Could you check a few things on this drawing? It's one solid part, dimensions in mm from its lowest x, y, z. Give positions to 0.01 mm unless a question says otherwise; leave off trailing zeros. Write each loop counter-clockwise with the first axis right and the second up, starting at its lowest first coordinate (ties: lowest second). Pieces come first, ordered by that corner, then holes.
1. Suppose I cut it at B-B (y = 74). Please give me the cut outline in (x, z).
2. If I drill on probe 1 along X at (y, z) = (28, 3); probe 2 along Y at (x, z) = (65.5, 5.25); probe 3 along X at (y, z) = (24, 3), over which ranges is the centre line in solid material (lowest first)?
3. I'm going to push flat-ended pins straight in: pin 1 (1.9 mm diameter, centred on y = 3, z = 2.5, fed in from +X); pin 2 (1.9 mm diameter, centred on y = 2.5, z = 3, fed in from -X); pin 3 (3 mm diameter, centred on y = 13, z = 3.5, fed in from -X). Where does each tip first touch, or does it pass through?
4. Suppose I cut it at A-A (x = 123). Please give me the cut outline in (y, z).
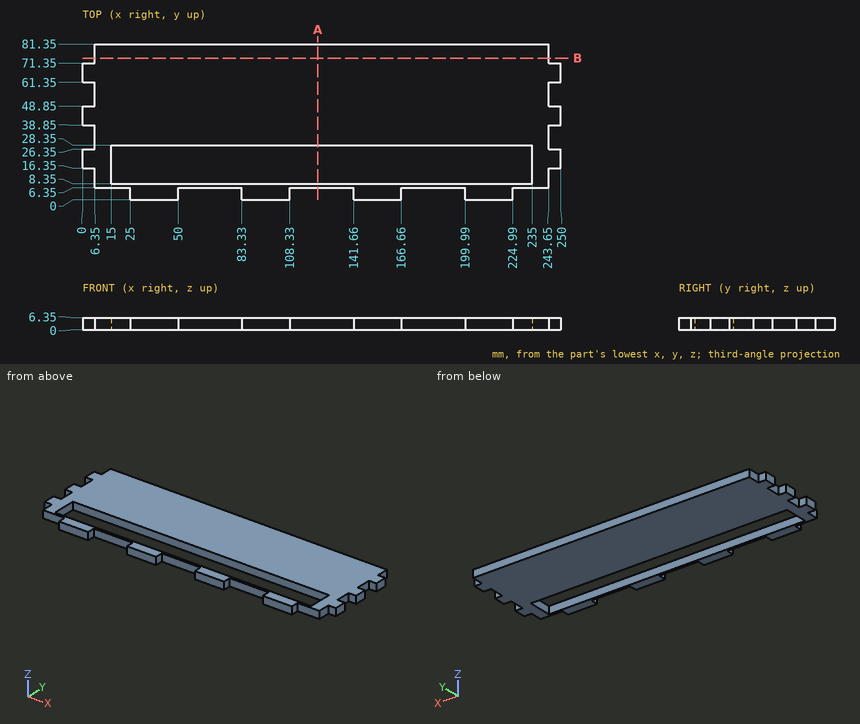
Checks:
1. outline: (6.35, 0) - (243.65, 0) - (243.65, 6.35) - (6.35, 6.35) - close
2. probe 1: x = 6.35 to 15, 235 to 243.65
2. probe 2: y = 6.35 to 8.35, 28.35 to 81.35
2. probe 3: x = 0 to 15, 235 to 250
3. pin 1: stops at x = 224.99
3. pin 2: stops at x = 25
3. pin 3: stops at x = 6.35
4. outline: (6.35, 0) - (8.35, 0) - (8.35, 6.35) - (6.35, 6.35) - close; (28.35, 0) - (81.35, 0) - (81.35, 6.35) - (28.35, 6.35) - close
